Here's the drawing with two shaded views (mm, measured from the low corner). I have some questions. A direction names the side the tool comes from. Round coordinates to 2 decimals unless told otherwise and drop trailing zeros. Loops run counter-clockwise (first coordinate to the right, second up) from the corner with the lowest first, then second, coordinate; pieces in that order, holes last.
(1) Which directions (+Z, -Z, +X, -X, +Y, -Y) give clear straight access to the entire face, cutting with the end or side of a thin tool? Please do the marked faces 1 and 2.
(2) I want a section at D-D on x = 7. Write out the boundary of the cut face in (y, z).
(3) I want a section at A-A on y = 20.5. Write out the boundary of the cut face in (x, z) (1 decimal).
(4) Thinking about a two-plate mould opening in Z: for the marked faces 3, 4, 5 and 6, which applies, released by +Z, released by -Z, zero draft, split by the parting line, or undercut?
(5) If I drill on line 1 along Z through (x, y) = (7.5, 33); line 2 along Y through (x, z) = (20.5, 14) (1 decimal); line 3 along Y through (x, z) = (24.5, 8) (1 decimal), over which ranges is the centre line in solid material (lowest first)?
(6) Will these pins go through, and if not, where does the flat tip stop? pin 1 Ø6 at (y, z) = (33.5, 15.5) entering from +X (1 decimal); pin 2 Ø6 at (x, z) = (14.5, 20.5) entering from -Y; pin 3 Ø6 at (y, z) = (11, 13.5) entering from -X.
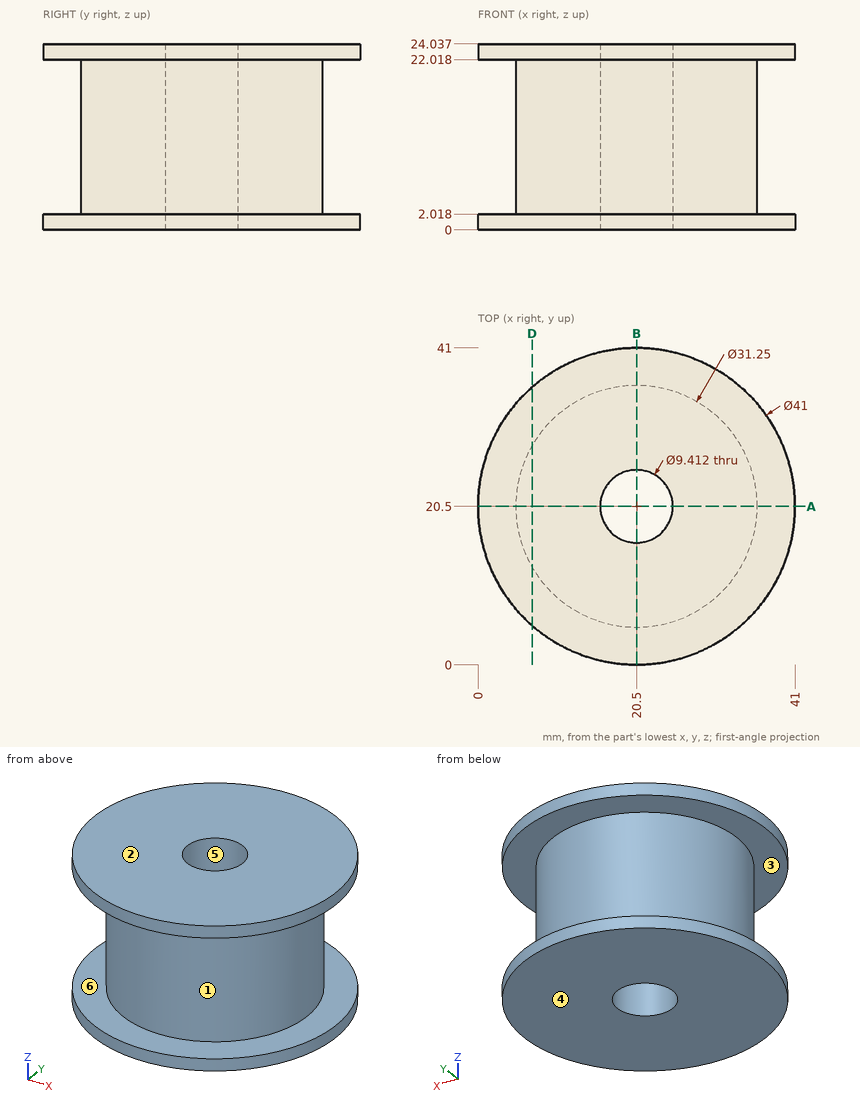
Filled sheet:
1. face 1: none
1. face 2: +Z, +X, -X, +Y, -Y
2. outline: (5.07, 0) - (35.93, 0) - (35.93, 2.02) - (28.37, 2.02) - (28.37, 22.02) - (35.93, 22.02) - (35.93, 24.04) - (5.07, 24.04) - (5.07, 22.02) - (12.63, 22.02) - (12.63, 2.02) - (5.07, 2.02) - close
3. outline: (0, 0) - (15.8, 0) - (15.8, 24) - (0, 24) - (0, 22) - (4.9, 22) - (4.9, 2) - (0, 2) - close; (25.2, 0) - (41, 0) - (41, 2) - (36.1, 2) - (36.1, 22) - (41, 22) - (41, 24) - (25.2, 24) - close
4. face 3: undercut
4. face 4: released by -Z
4. face 5: zero draft
4. face 6: undercut
5. line 1: z = 0 to 2.02, 22.02 to 24.04
5. line 2: y = 4.9 to 15.8, 25.2 to 36.1
5. line 3: y = 5.4 to 18, 23 to 35.6
6. pin 1: stops at x = 32.5
6. pin 2: stops at y = 0.29
6. pin 3: stops at x = 6.29
